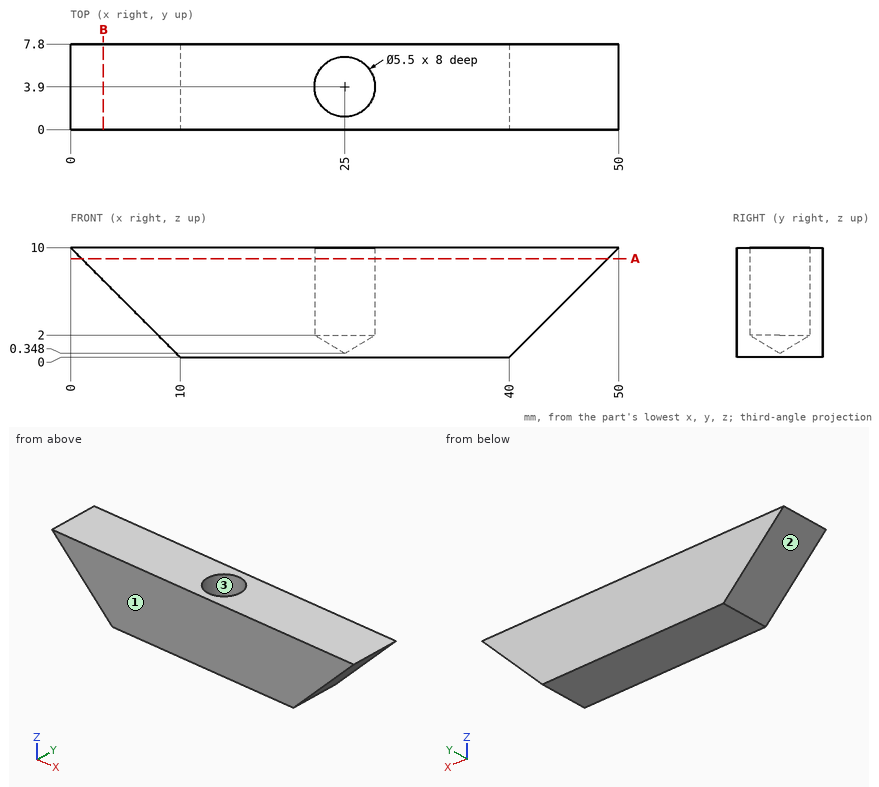
Study the drawing (mm; zero at the part's minimum x, y, z) and answer. Coordinates: 2 decimals unless noted, no trailing zeros. Write each loop counter-clockwise with the first axis right and the second up, starting at its lowest first coordinate (ties: lowest second). Pieces come first, ordered by that corner, then holes. Notation, with made-up numbers: (62.5, -14.75) - (68.5, -14.75) arc R25 cw to (68.5, 0.25) - close; hole circle Ø4 at (64.25, 68.5). An arc over 180 degrees is marked (long way). Put each result on its own line as item: value.
1. The part is cut by section B-B on x = 3. Give the vertices of the cut face in (y, z), plus the area to 3 significant figures.
Answer sheet:
outline: (0, 7) - (7.8, 7) - (7.8, 10) - (0, 10) - close
area: 23.4 mm^2
2. Find the intervals of material crossed by line 1 along Y through (x, z) = (25, 4); line 2 along X through (y, z) = (3.9, 4.75); line 3 along X through (y, z) = (3.9, 7.5), in increasing order. Write a range as from..to.
Answer sheet:
line 1: y = 0..1.15, 6.65..7.8
line 2: x = 5.25..22.25, 27.75..44.75
line 3: x = 2.5..22.25, 27.75..47.5
3. The part is cut by section A-A on z = 9. Give the vertices of the cut face in (x, y), plus the area to 3 significant figures.
Answer sheet:
outline: (1, 0) - (49, 0) - (49, 7.8) - (1, 7.8) - close; hole circle Ø5.5 at (25, 3.9)
area: 351 mm^2
4. A flat-ended cylindrical pin translates along its axis: pin 1 Ø1 at (y, z) = (2, 3) entering from -X. Find the tip coordinate at first contact, or state that the pin passes through.
Answer sheet:
pin 1: stops at x = 6.5
5. Determine the mould class of the marked faces 1, 2 and 3 for opening direction X: pulls with the +X half, pulls with the -X half, needs draft (parallel to the pull), parting line crosses it, or undercut.
Answer sheet:
face 1: needs draft
face 2: pulls with the -X half
face 3: undercut
